```python
from build123d import *

# Parameters (mm, degrees)
BOSS_EXTRU_1_DEPTH      = 1.6
ENL_V_MAT_EXTRU_1_REACH = 29.149
ESQUISSE2_R             = 1


with BuildPart() as part:
    # Esquisse1 → Boss.-Extru.1 (new body)
    with BuildSketch(Plane(origin=(0, 0, 0), x_dir=(1, 0, 0), z_dir=(0, 1, 0))):
        with BuildLine():
            Line((-20.5, -16.5), (20.5, -16.5))
            ThreePointArc((20.5, -16.5), (21.207106781, -16.207106781), (21.5, -15.5))
            Line((21.5, -15.5), (21.5, 15.5))
            ThreePointArc((21.5, 15.5), (21.207106781, 16.207106781), (20.5, 16.5))
            Line((20.5, 16.5), (-20.5, 16.5))
            ThreePointArc((-20.5, 16.5), (-21.207106781, 16.207106781), (-21.5, 15.5))
            Line((-21.5, 15.5), (-21.5, -15.5))
            ThreePointArc((-21.5, -15.5), (-21.207106781, -16.207106781), (-20.5, -16.5))
        make_face()
    extrude(amount=BOSS_EXTRU_1_DEPTH)

    # Esquisse2 → Enlèv. mat.-Extru.1 (cut, up to next)
    with BuildSketch(Plane(origin=(0, 1.6, 0), x_dir=(1, 0, 0), z_dir=(0, 1, 0)), mode=Mode.PRIVATE) as enl_v_mat_extru_1_sk1:
        with Locations(Location((-14.5, 13.75, 0), (0, 0, 270))):
            Circle(ESQUISSE2_R)
    enl_v_mat_extru_1_tool1 = extrude(enl_v_mat_extru_1_sk1.sketch, amount=-ENL_V_MAT_EXTRU_1_REACH, mode=Mode.PRIVATE) & part.part
    # Esquisse2 → Enlèv. mat.-Extru.1 (cut, up to next)
    with BuildSketch(Plane(origin=(0, 1.6, 0), x_dir=(1, 0, 0), z_dir=(0, 1, 0)), mode=Mode.PRIVATE) as enl_v_mat_extru_1_sk2:
        with Locations(Location((14.5, 13.75, 0), (0, 0, 270))):
            Circle(ESQUISSE2_R)
    enl_v_mat_extru_1_tool2 = extrude(enl_v_mat_extru_1_sk2.sketch, amount=-ENL_V_MAT_EXTRU_1_REACH, mode=Mode.PRIVATE) & part.part
    # Esquisse2 → Enlèv. mat.-Extru.1 (cut, up to next)
    with BuildSketch(Plane(origin=(0, 1.6, 0), x_dir=(1, 0, 0), z_dir=(0, 1, 0)), mode=Mode.PRIVATE) as enl_v_mat_extru_1_sk3:
        with Locations(Location((14.5, -13.75, 0), (0, 0, 270))):
            Circle(ESQUISSE2_R)
    enl_v_mat_extru_1_tool3 = extrude(enl_v_mat_extru_1_sk3.sketch, amount=-ENL_V_MAT_EXTRU_1_REACH, mode=Mode.PRIVATE) & part.part
    # Esquisse2 → Enlèv. mat.-Extru.1 (cut, up to next)
    with BuildSketch(Plane(origin=(0, 1.6, 0), x_dir=(1, 0, 0), z_dir=(0, 1, 0)), mode=Mode.PRIVATE) as enl_v_mat_extru_1_sk4:
        with Locations(Location((-14.5, -13.75, 0), (0, 0, 270))):
            Circle(ESQUISSE2_R)
    enl_v_mat_extru_1_tool4 = extrude(enl_v_mat_extru_1_sk4.sketch, amount=-ENL_V_MAT_EXTRU_1_REACH, mode=Mode.PRIVATE) & part.part
    add(enl_v_mat_extru_1_tool1.solids().sort_by_distance((-14.5, 1.6, -13.75))[0], mode=Mode.SUBTRACT)
    add(enl_v_mat_extru_1_tool2.solids().sort_by_distance((14.5, 1.6, -13.75))[0], mode=Mode.SUBTRACT)
    add(enl_v_mat_extru_1_tool3.solids().sort_by_distance((14.5, 1.6, 13.75))[0], mode=Mode.SUBTRACT)
    add(enl_v_mat_extru_1_tool4.solids().sort_by_distance((-14.5, 1.6, 13.75))[0], mode=Mode.SUBTRACT)


solid = part.part
```
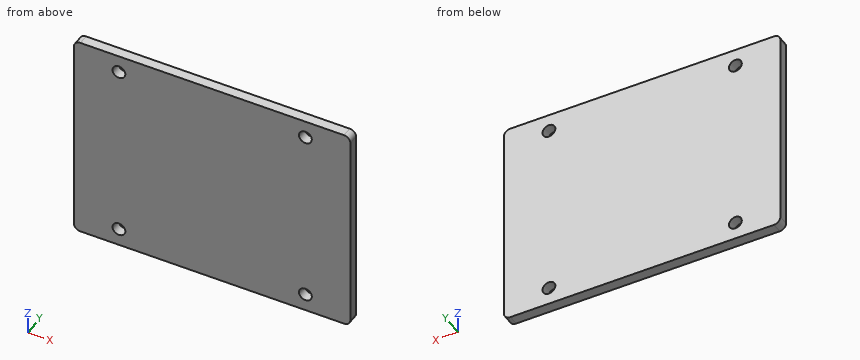
Verification items for the finished model (mm, model axes). Give positions to 0.01 mm unless a question says otherwise; leave off trailing zeros. Write each loop counter-clockwise with the first axis right and the second up, starting at its lowest first coordinate (ties: lowest second). Pieces come first, ordered by that corner, then holes. Notation, with made-up numbers: (86.25, 25) - (122.25, 25) arc R15 cw to (122.25, 41) - close; hole circle Ø6 at (68.5, 69). An arc over 180 degrees is marked (long way). Put each result on its own line as item: value.
Q1. Scan lines: probe 1 along X at (y, z) = (0.95, 13.75); probe 2 along Z at (x, y) = (15, 1.2); probe 3 along X at (y, z) = (1.1, -13). Record each from-to range of solid material in increasing order. Write a range as from..to.
Result:
probe 1: -21.5..-15.5, -13.5..13.5, 15.5..21.5
probe 2: -16.5..-14.62, -12.88..12.88, 14.62..16.5
probe 3: -21.5..-15.16, -13.84..13.84, 15.16..21.5
Q2. Section check A-A on x = 14.5. Record the cut outline in (y, z).
Result:
outline: (0, -16.5) - (1.6, -16.5) - (1.6, -14.75) - (0, -14.75) - close; (0, -12.75) - (1.6, -12.75) - (1.6, 12.75) - (0, 12.75) - close; (0, 14.75) - (1.6, 14.75) - (1.6, 16.5) - (0, 16.5) - close
Q3. Depth check by flat-ended pin: P1, Ø1.6, axis at x = -14.5, z = 13.75, coming from the -Y side; P2, Ø8, axis at x = -13.5, z = -0.5, coming from the -Y side. Enter the tip coordinate at first touch or a pass-through.
Result:
P1: through
P2: y = 0
Q4. Section check B-B on z = 13.75. Record the cut outline in (x, y).
Result:
outline: (-21.5, 0) - (-15.5, 0) - (-15.5, 1.6) - (-21.5, 1.6) - close; (-13.5, 0) - (13.5, 0) - (13.5, 1.6) - (-13.5, 1.6) - close; (15.5, 0) - (21.5, 0) - (21.5, 1.6) - (15.5, 1.6) - close
